Geometry: final body of the model. Coordinates: model frame, mm. A direction names the side the tool comes from. Give positions to 0.01 mm unless a question says otherwise; leave off trailing zeros. Write each loop counter-clockwise with the first axis right and the second up, starting at its lowest first coordinate (ties: lowest second). Pieces come first, ordered by that corner, then holes.
```python
from build123d import *

# Parameters (mm, degrees)
F0_W     = 127.7336031199
F0_H     = 117.6951080561
F1_DEPTH = 25.4
F2_R     = 25.4
F4_DEPTH = 8
F6_DEPTH = 25.4
F6_TAPER = 6


with BuildPart() as f1:
    # F0 (on Top) → F1 (new body)
    with BuildSketch(Plane.XY):
        with Locations((63.8668015599, 58.847554028)):
            Rectangle(F0_W, F0_H)
    extrude(amount=F1_DEPTH)

    # F2
    f2_edges = [f1.edges().sort_by_distance(p)[0] for p in [
        (127.733603, 117.695108, 12.7),
    ]]
    fillet(f2_edges, radius=F2_R)

    # F3 (on face) → F4 (cut)
    with BuildSketch(Plane.XY.offset(25.4)):
        with BuildLine():
            ThreePointArc((38.8666712233, 28.4028087029), (76.3769148887, 58.9921224705), (27.9881136193, 57.8748005294))
            ThreePointArc((27.9881136193, 57.8748005294), (22.7769180991, 39.2075535793), (38.8666712233, 28.4028087029))
        make_face()
    extrude(amount=-F4_DEPTH, mode=Mode.SUBTRACT)

    # F5 (on face) → F6 (join)
    with BuildSketch(Plane.XY.offset(25.4)):
        with BuildLine():
            ThreePointArc((77.0522903969, 94.7477040289), (91.3384484979, 83.0158556177), (100.5024355694, 66.9612014208))
            ThreePointArc((100.5024355694, 66.9612014208), (119.6345907249, 73.6984463156), (127.7336031199, 92.2951080561))
            ThreePointArc((127.7336031199, 92.2951080561), (120.294115362, 110.2556202982), (102.3336031199, 117.6951080561))
            ThreePointArc((102.3336031199, 117.6951080561), (85.26222265, 111.1027652428), (77.0522903969, 94.7477040289))
        make_face()
    extrude(amount=F6_DEPTH, taper=F6_TAPER)


solid = f1.part
```
Item 1: Reachability of faces 5 (the face through (50, 117.695, 13)), 6 (the face through (76.67, 58.15, 21.46)) from +Z, -Z, +X, -X, +Y, -Y: full face, straight path, thin tool, end or side. Return the list, or none.
Found:
face 5: +Z, -Z, +X, -X, +Y
face 6: +Z
Item 2: Pin query (flat end, axial travel): pin 1 Ø12 at (x, y) = (101, 102) entering from -Z; pin 2 Ø5 at (x, y) = (33, 77) entering from +Z; pin 3 Ø12 at (x, z) = (112, 45) entering from +Y; pin 4 Ø4 at (x, z) = (106, 29.5) entering from +Y. Return the tip coordinate at first contact, or that it passes through.
Found:
pin 1: stops at z = 0
pin 2: stops at z = 25.4
pin 3: stops at y = 115.52
pin 4: stops at y = 117.31
Item 3: Section A-A, the plane y = 12. Return the cut outline in (x, z).
Found:
outline: (0, 0) - (127.73, 0) - (127.73, 25.4) - (0, 25.4) - close
Item 4: Line query: L1, parallel to Z at x = 42, y = 56; L2, parallel to Z at x = 93.5, y = 48; L3, parallel to X at y = 66.5, z = 24. Output: solid intervals per line, ascending.
Found:
L1: z = 0 to 17.4
L2: z = 0 to 25.4
L3: x = 0 to 32.71, 72.04 to 127.73
Item 5: Section B-B, the plane x = 72. Return the cut outline in (y, z), plus the area to 3 significant figures.
Found:
outline: (0, 0) - (117.7, 0) - (117.7, 25.4) - (66.55, 25.4) - (66.55, 17.4) - (33.72, 17.4) - (33.72, 25.4) - (0, 25.4) - close
area: 2,730 mm2
Item 6: Pull-direction query (X, two-part tool) for faces 1 (the face through (22.68, 39.48, 21.46)), 2 (the face through (63, 60, 0)), 3 (the face through (49, 50, 17.4)), 4 (the face through (120.49, 110.06, 12.88)); classes: +X half, -X half, draft (parallel to the pull), parting line (faces both ways), or undercut.
Found:
face 1: undercut
face 2: draft
face 3: undercut
face 4: +X half
